Autodesk Inventor part; units mm, degrees
ref_plane "YZ Plane" through (0, 0, 0) normal (1, 0, 0) x (0, 1, 0)
ref_plane "XZ Plane" through (0, 0, 0) normal (0, 1, 0) x (-1, 0, 0)
ref_plane "XY Plane" through (0, 0, 0) normal (0, 0, 1) x (1, 0, 0)
sketch "Sketch1" plane through (0, 0, 0) normal (1, 0, 0) x (0, 1, 0)
  line L0 (0, 0) -> (10, 0)
  line L1 (10, 0) -> (10, -10)
  line L2 (10, -10) -> (0, -10)
  line L3 (0, -10) -> (0, 0)
  dimension "d0" = 10
  dimension "d1" = 10
extrude "Extrusion1" add sketch "Sketch1" along normal blind 10
sketch "Sketch4" plane through (0, 0, 0) normal (0, 0, 1) x (1, 0, 0)
  line L0 (1.8731, 7.9408) -> (4.4271, 7.9408) construction
  line L1 (4.4271, 7.9408) -> (4.4271, 4.8928) construction
  line L2 (4.4271, 4.8928) -> (1.8731, 4.8928) construction
  line L3 (1.8731, 4.8928) -> (1.8731, 7.9408) construction
  spline S0 degree 2 poles (6.7794, 4.2913) (6.548, 3.1344) (5.0493, 1.7514) (4.0292, 1.7514) knots 0 0 0 1 2 2 2
  spline S1 degree 2 poles (4.0292, 1.7514) (3.0984, 1.7514) (2.1729, 2.7873) (2.1729, 3.8285) knots 0 0 0 1 2 2 2
  spline S2 degree 2 poles (2.1729, 3.8285) (2.1729, 4.8066) (3.0984, 6.8785) (3.8241, 7.5148) knots 0 0 0 1 2 2 2
  spline S3 degree 2 poles (3.8241, 7.5148) (4.3079, 7.9408) (4.8442, 7.9408) knots 0 0 0 1 1 1
  spline S4 degree 2 poles (4.8442, 7.9408) (5.1861, 7.9408) (5.7487, 7.7146) knots 0 0 0 1 1 1
  spline S5 degree 2 poles (5.7487, 7.7146) (6.4376, 7.4412) (6.4376, 7.1152) knots 0 0 0 1 1 1
  spline S6 degree 2 poles (6.4376, 7.1152) (6.4376, 6.9574) (6.2115, 6.7155) (6.0537, 6.7155) knots 0 0 0 1 2 2 2
  spline S7 degree 2 poles (6.0537, 6.7155) (5.9696, 6.7155) (5.8171, 6.8102) knots 0 0 0 1 1 1
  spline S8 degree 2 poles (5.8171, 6.8102) (5.2439, 7.1625) (4.8442, 7.1625) knots 0 0 0 1 1 1
  spline S9 degree 2 poles (4.8442, 7.1625) (4.5603, 7.1625) (4.25, 6.868) knots 0 0 0 1 1 1
  spline S10 degree 2 poles (4.25, 6.868) (4.0975, 6.7208) (3.8083, 6.3316) knots 0 0 0 1 1 1
  spline S11 degree 2 poles (3.8083, 6.3316) (2.9354, 5.18) (2.9354, 3.8285) knots 0 0 0 1 1 1
  spline S12 degree 2 poles (2.9354, 3.8285) (2.9354, 3.1186) (3.1562, 2.8346) knots 0 0 0 1 1 1
  spline S13 degree 2 poles (3.1562, 2.8346) (3.3929, 2.5244) (4.0292, 2.5244) knots 0 0 0 1 1 1
  spline S14 degree 2 poles (4.0292, 2.5244) (4.7023, 2.5244) (5.2018, 2.9503) knots 0 0 0 1 1 1
  spline S15 degree 2 poles (5.2018, 2.9503) (5.7277, 3.4026) (5.9328, 4.2439) knots 0 0 0 1 1 1
  spline S16 degree 2 poles (5.9328, 4.2439) (4.8916, 4.1914) (4.1448, 3.8443) knots 0 0 0 1 1 1
  spline S17 degree 2 poles (4.1448, 3.8443) (4.0554, 3.8022) (3.9766, 3.8022) knots 0 0 0 1 1 1
  spline S18 degree 2 poles (3.9766, 3.8022) (3.8083, 3.8022) (3.6979, 3.9284) knots 0 0 0 1 1 1
  spline S19 degree 2 poles (3.6979, 3.9284) (3.5979, 4.0494) (3.5979, 4.2019) knots 0 0 0 1 1 1
  spline S20 degree 2 poles (3.5979, 4.2019) (3.5979, 4.407) (3.7978, 4.5332) knots 0 0 0 1 1 1
  spline S21 degree 2 poles (3.7978, 4.5332) (4.6129, 5.0275) (6.6059, 5.0275) knots 0 0 0 1 1 1
  spline S22 degree 2 poles (6.6059, 5.0275) (6.7636, 5.0275) (6.9845, 4.8066) (6.9845, 4.6436) knots 0 0 0 1 2 2 2
  spline S23 degree 2 poles (6.9845, 4.6436) (6.9845, 4.3964) (6.7794, 4.2913) knots 0 0 0 1 1 1
  point P0 (0, 0)
extrude "Extrusion4" cut sketch "Sketch4" against normal blind 2
sketch "Sketch5" plane through (10, 0, 0) normal (1, 0, 0) x (0, 0, -1)
  line L0 (3.1, 3.1) -> (6.2, 3.1)
  line L1 (6.2, 3.1) -> (6.2, 6.2)
  line L2 (6.2, 6.2) -> (3.1, 6.2)
  line L3 (3.1, 6.2) -> (3.1, 3.1)
  point P0 (0, 0)
  dimension "d11" = 3.1
  dimension "d12" = 3.1
extrude "Extrusion5" add sketch "Sketch5" along normal blind 5
properties part number "Guanine"
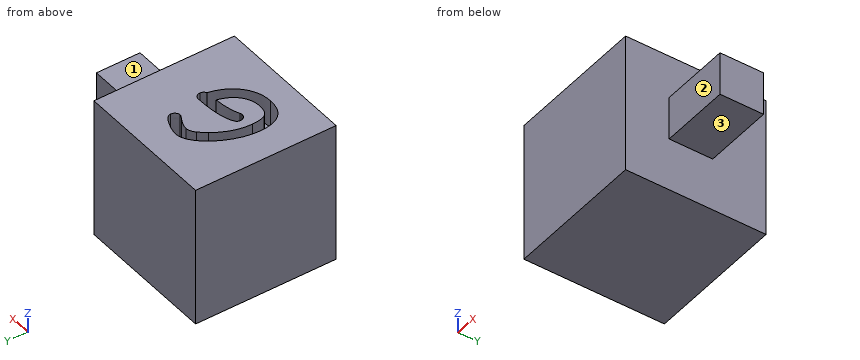
Verification items for the finished model (mm, model axes). Face numbers are marked on the shaded views. A direction names the side the tool comes from. Give positions to 0.01 mm unless a question says otherwise; leave off trailing zeros. Loops run counter-clockwise (first coordinate to the right, second up) from the corner with the lowest first, then second, coordinate; pieces in that order, holes last. Notation, with made-up numbers: (56, 78) - (84, 78) arc R12 ccw to (84, 84) - close; hole circle Ø2 at (23.25, 29.25). An arc over 180 degrees is marked (long way). Write item = value, one per line. Start each with the question number.
Q1. Tool access check on the marked faces 1, 2 and 3. Record the directions out of +Z, -Z, +X, -X, +Y, -Y that give a thin tool (end or side, any length) a straight path to the whole face; none if there is none.
Q2. Cross-section at B-B, the plane x = 11.5. Enter the section's corners in (y, z).
Q3. Thickness scan on line 1 (X direction, y = 7.5, z = -9); line 2 (Y direction, x = 6, z = -1); line 3 (Z direction, x = 2.25, y = 4.25). Record the ranges inside material, lowest first.
Q4. Cross-section at C-C, the plane y = 1.5. Enter the section's corners in (x, z), and give its area (3 significant figures).
Q5. Depth check by flat-ended pin: P1, Ø0.9, axis at x = 13.5, z = -4.5, coming from the -Y side; P2, Ø0.9, axis at x = 12, y = 4, coming from the -Z side; P3, Ø0.9, axis at x = 13, z = -4, coming from the +Y side. Enter the tip coordinate at first touch or a pass-through.
Q6. Cross-section at A-A, the plane z = -3.5. Enter the section's corners in (x, y), and give its area (4 significant figures).
Answer key:
q1.face_1 = +Z, +X, +Y, -Y
q1.face_2 = +Z, -Z, +X, -Y
q1.face_3 = -Z, +X, +Y, -Y
q2.outline = (3.1, -6.2) - (6.2, -6.2) - (6.2, -3.1) - (3.1, -3.1) - close
q3.line_1 = 0 to 10
q3.line_2 = 0 to 2.65, 5.01 to 6.72, 7.6 to 10
q3.line_3 = -10 to -2
q4.outline = (0, -10) - (10, -10) - (10, 0) - (0, 0) - close
q4.area = 100 mm^2
q5.P1 = 3.1
q5.P2 = -6.2
q5.P3 = 6.2
q6.outline = (0, 0) - (10, 0) - (10, 3.1) - (15, 3.1) - (15, 6.2) - (10, 6.2) - (10, 10) - (0, 10) - close
q6.area = 115.5 mm^2
